Read the model definition and answer for the solid it produces. Units are mm, in the model's axes. Coordinates: 2 decimals unless noted, no trailing zeros. Write each loop counter-clockwise with the first axis right and the second up, starting at its lowest first coordinate (ties: lowest second). Pieces come first, ordered by that corner, then holes.
(1) Section A-A on z = 1.85 is taken. Write down the section's boundary in (x, y).
(2) Given pin 1 (0.9 mm diameter, centred on y = 48, z = 1, fed in from +X); pin 2 (1.5 mm diameter, centred on y = 44.5, z = 0.5, fed in from +X); pin 3 (1.5 mm diameter, centred on x = 42, z = 2, fed in from +Y); pin 4 (10 mm diameter, centred on x = 44.5, y = 20.5, fed in from -Z), each flat-ended and moving along its own axis, determine where each tip first touches the part or whether it passes through.
(3) Section B-B on x = 48.5 is taken. Write down the section's boundary in (y, z).
(4) Section C-C on y = 6.5 is taken. Write down the section's boundary in (x, z).
(5) Find the intervals of material crossed by probe 1 along X at (y, z) = (47.5, 2.8); probe 2 along X at (y, z) = (9.5, 2.55); probe 3 along Y at (x, z) = (41, 2.25), in increasing order.
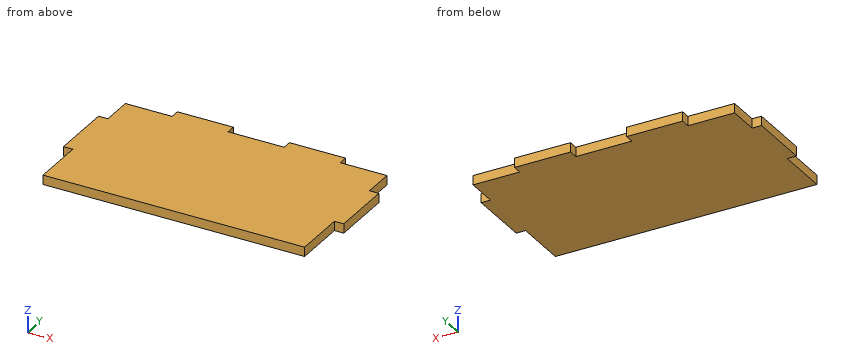
from build123d import *

# Parameters (mm, degrees)
SKETCH1_W           = 90
SKETCH1_H           = 50
BOSS_EXTRUDE1_DEPTH = 3
SKETCH2_W           = 18
SKETCH2_H           = 3
SKETCH2_W_2         = 3
SKETCH2_H_2         = 17
CUT_EXTRUDE1_DEPTH  = 3


with BuildPart() as part:
    # Sketch1 → Boss-Extrude1 (new body)
    with BuildSketch(Plane.XY):
        with Locations((45, 25)):
            Rectangle(SKETCH1_W, SKETCH1_H)
    extrude(amount=BOSS_EXTRUDE1_DEPTH)

    # Sketch2 → Cut-Extrude1 (cut)
    with BuildSketch(Plane.XY.offset(3)):
        Polygon((0, 50), (18, 50), (18, 47), (3, 47), (3, 37), (0, 37), (0, 47), align=None)
        with Locations((45, 48.5)):
            Rectangle(SKETCH2_W, SKETCH2_H)
        Polygon((90, 50), (72, 50), (72, 47), (87, 47), (87, 37), (90, 37), (90, 47), align=None)
        with Locations((88.5, 8.5)):
            Rectangle(SKETCH2_W_2, SKETCH2_H_2)
        with Locations((1.5, 8.5)):
            Rectangle(SKETCH2_W_2, SKETCH2_H_2)
    extrude(amount=-CUT_EXTRUDE1_DEPTH, mode=Mode.SUBTRACT)


solid = part.part
Response:
1. outline: (0, 17) - (3, 17) - (3, 0) - (87, 0) - (87, 17) - (90, 17) - (90, 37) - (87, 37) - (87, 47) - (72, 47) - (72, 50) - (54, 50) - (54, 47) - (36, 47) - (36, 50) - (18, 50) - (18, 47) - (3, 47) - (3, 37) - (0, 37) - close
2. pin 1: stops at x = 72
2. pin 2: stops at x = 87
2. pin 3: stops at y = 47
2. pin 4: stops at z = 0
3. outline: (0, 0) - (47, 0) - (47, 3) - (0, 3) - close
4. outline: (3, 0) - (87, 0) - (87, 3) - (3, 3) - close
5. probe 1: x = 18 to 36, 54 to 72
5. probe 2: x = 3 to 87
5. probe 3: y = 0 to 47
